Model file for the job. Use its own axes, mm. A direction names the side the tool comes from. Coordinates: 2 decimals unless noted, no trailing zeros. Order: outer loops, then holes, each group sorted by start corner. A loop starts at its lowest first (then second) coordinate and runs counter-clockwise, first axis right, second up. Notation, with made-up numbers: (-7, 7) -> (0, 7) arc R21 cw to (0, 16) -> close; hole circle Ø9 at (-10.75, 69.25). An arc over 180 degrees is marked (long way). Use CSV: the item, a comma, the result in double quotes. Start each with the question number.
(1) Cut at D-D on z = 7.5. Write the cut outline in (x, y), plus the area to 3 significant figures.
(2) Cut at C-C on z = 35.5. Write the cut outline in (x, y), plus the area to 3 significant figures.
(3) Tool access for faces 1 (the cylindrical face through (3.05, -1.26, 34.52)), 2 (the flat face through (5, -4.762, 3)), 3 (the flat face through (0, 0, 2.54)): list every direction of +Z, -Z, +X, -X, +Y, -Y with a clear straight run to the whole face (end or side of a thin tool).
(4) Pin check, flat tips, straight feed: pin 1 Ø10 at (x, z) = (12.5, 18.5) entering from -Y; pin 2 Ø5 at (x, y) = (13, 2.5) entering from +Z; pin 3 Ø5 at (y, z) = (-3, 20) entering from +X. Stop position of each tip, or through.
(5) Probe L1, parallel to Y at x = 0, z = 1.35; L2, parallel to Z at x = -3.75, y = 0; L3, parallel to Y at x = -0.25, z = 44. List the from-to ranges inside material, lowest first.
(6) Cut at A-A on y = 0. Write the cut outline in (x, z), plus the area to 3 significant figures.
(7) Cut at B-B on x = 0. Write the cut outline in (y, z), plus the area to 3 significant figures.
(8) Pull direction Y, two halves, no side cores. Call faces 4 (the cylindrical face through (-6.35, 0.1, 3.13)), 5 (the flat face through (5, 0, 6.35)), 6 (the cylindrical face through (10.94, -0.49, 1.25)): pulls with the +Y half, pulls with the -Y half, needs draft (parallel to the pull), parting line crosses it, or undercut.
```python
from build123d import *

# Parameters (mm, degrees)
F1_DEPTH = 63.5
F0_R     = 3.302
F2_DEPTH = 19.05
F3_DEPTH = 5.08
F4_DEPTH = 1.27
F5_R     = 3.302
F6_R     = 1.27
F7_DEPTH = 2.54


with BuildPart() as f1:
    # F0 (on Top) → F1 (new body)
    with BuildSketch(Plane.XY):
        with BuildLine():
            ThreePointArc((-3.302, 0), (0, -3.302), (3.302, 0))
            ThreePointArc((3.302, 0), (0, 3.302), (-3.302, 0))
        make_face()
    extrude(amount=F1_DEPTH)



with BuildPart() as f2:
    # F0 (on Top) → F2 (new body)
    with BuildSketch(Plane.XY):
        with Locations((9.8069049418, 0)):
            Circle(F0_R)
    extrude(amount=F2_DEPTH)


with BuildPart() as f1_1:
    add(f1.part)

    add(f2.part)  # F3 merges F2
    # F0 (on Top) → F3 (join)
    with BuildSketch(Plane.XY):
        with BuildLine():
            Line((11.3944049418, 4.7625), (-1.5875, 4.7625))
            ThreePointArc((-1.5875, 4.7625), (-6.35, 0), (-1.5875, -4.7625))
            Line((-1.5875, -4.7625), (11.3944049418, -4.7625))
            ThreePointArc((11.3944049418, -4.7625), (16.1569049418, 0), (11.3944049418, 4.7625))
        make_face()
        with BuildLine():
            ThreePointArc((-3.302, 0), (0, 3.302), (3.302, 0))
            ThreePointArc((3.302, 0), (0, -3.302), (-3.302, 0))
        make_face(mode=Mode.SUBTRACT)
        with Locations((9.8069049418, 0)):
            Circle(F0_R, mode=Mode.SUBTRACT)
    extrude(amount=F3_DEPTH)

    # F4 (add): a face of the model
    f4_faces = [f1_1.faces().sort_by_distance(p)[0] for p in [
        (4.9034524709, 0, 5.08),
    ]]
    extrude(f4_faces, amount=F4_DEPTH)

    # F5
    f5_edges = [f1_1.edges().sort_by_distance(p)[0] for p in [
        (6.504905, 0, 19.05),
    ]]
    fillet(f5_edges, radius=F5_R)

    # F6 (on face) → F7 (cut)
    with BuildSketch(Plane.XY):
        Circle(F6_R)
        with Locations((9.7663812339, 0)):
            Circle(F6_R)
    extrude(amount=F7_DEPTH, mode=Mode.SUBTRACT)


solid = f1_1.part
```
Outcome:
1,outline,"circle Ø6.6 at (0, 0); circle Ø6.6 at (9.81, 0)"
1,area,"68.5 mm2"
2,outline,"circle Ø6.6 at (0, 0)"
2,area,"34.3 mm2"
3,face 1,"+Z"
3,face 2,"+Z, -Z, +X, -X, -Y"
3,face 3,"-Z"
4,pin 1,"y = -3.3"
4,pin 2,"z = 18.66"
4,pin 3,"x = 11.7"
5,L1,"-4.76 to -1.27, 1.27 to 4.76"
5,L2,"0 to 6.35"
5,L3,"-3.29 to 3.29"
6,outline,"(-6.35, 0) -> (-1.27, 0) -> (-1.27, 2.54) -> (1.27, 2.54) -> (1.27, 0) -> (8.5, 0) -> (8.5, 2.54) -> (11.04, 2.54) -> (11.04, 0) -> (16.16, 0) -> (16.16, 6.35) -> (13.11, 6.35) -> (13.11, 15.75) arc R3.3 ccw to (6.5, 15.75) -> (6.5, 6.35) -> (3.3, 6.35) -> (3.3, 63.5) -> (-3.3, 63.5) -> (-3.3, 6.35) -> (-6.35, 6.35) -> close"
6,area,"587 mm2"
7,outline,"(-4.76, 0) -> (-1.27, 0) -> (-1.27, 2.54) -> (1.27, 2.54) -> (1.27, 0) -> (4.76, 0) -> (4.76, 6.35) -> (3.3, 6.35) -> (3.3, 63.5) -> (-3.3, 63.5) -> (-3.3, 6.35) -> (-4.76, 6.35) -> close"
7,area,"431 mm2"
8,face 4,"parting line crosses it"
8,face 5,"needs draft"
8,face 6,"undercut"
